Build history of the part. All positions in model axes, mm. A direction names the side the tool comes from. Round coordinates to 2 decimals unless told otherwise and drop trailing zeros. Write each loop counter-clockwise with the first axis right and the second up, starting at its lowest first coordinate (ties: lowest second). Pieces come first, ordered by that corner, then holes. Notation, with made-up numbers: (38.25, 2.25) -> (97.25, 2.25) arc R11 ccw to (97.25, 12.25) -> close; hole circle Ø11 at (20, 66). An arc over 180 degrees is marked (long way). One line per question, with ' | ' between items.
from build123d import *

# Parameters (mm, degrees)
F_3_6_3_6_DIAMETER_HOLE1_D     = 3.6
F_3_6_3_6_DIAMETER_HOLE1_DEPTH = 12
F_3_6_3_6_DIAMETER_HOLE1_TIP   = 1.081549114


with BuildPart() as part:
    # Sketch1 → Revolve1 (revolve)
    with BuildSketch(Plane.XY, mode=Mode.PRIVATE) as revolve1_sk:
        with BuildLine():
            Line((0, 14.67), (0, 5.5))
            Line((0, 5.5), (27, 5.5))
            Line((27, 5.5), (27, 11))
            ThreePointArc((27, 11), (22.050252532, 13.050252532), (20, 18))
            Line((20, 18), (20, 20))
            ThreePointArc((20, 20), (16, 24), (12, 20))
            Line((12, 20), (11, 20))
            Line((11, 20), (11, 13.17))
            Line((11, 13.17), (8, 13.17))
            Line((8, 13.17), (8, 14.67))
            Line((8, 14.67), (0, 14.67))
        make_face()
    revolve(revolve1_sk.sketch.rotate(Axis((0, 0, 0), (1, 0, 0)), 90), axis=Axis((0, 0, 0), (1, 0, 0)))

    # Ø3.6 (3.6) Diameter Hole1
    with Locations(Plane(origin=(21.47261693, 9.449479998, -9.92628458), x_dir=(0.49047083458, 0, 0.871457606787), z_dir=(0.789626152924, 0.423067471154, -0.444414731382))):
        with Locations((0, 0)):
            Hole(F_3_6_3_6_DIAMETER_HOLE1_D / 2, depth=F_3_6_3_6_DIAMETER_HOLE1_DEPTH)
            with Locations((0, 0, -(F_3_6_3_6_DIAMETER_HOLE1_DEPTH + F_3_6_3_6_DIAMETER_HOLE1_TIP / 2))):  # 118° drill point
                Cone(0, F_3_6_3_6_DIAMETER_HOLE1_D / 2, F_3_6_3_6_DIAMETER_HOLE1_TIP, mode=Mode.SUBTRACT)


solid = part.part
(1) Wall check: line 1 (Y direction, x = 16, z = 0); line 2 (Y direction, x = 7, z = 0); line 3 (X direction, y = 13.5, z = -5). Give the ranges that are in metal, low to high. Write a range as from..to.
Calculated:
line 1: -24..-5.5, 5.5..24 | line 2: -14.67..-5.5, 5.5..14.67 | line 3: 0..8, 11..21
(2) Slice it at A-A (z = 0). Write the cut outline in (x, y), then the cut area to 3 significant figures.
Calculated:
outline: (0, -14.67) -> (8, -14.67) -> (8, -13.17) -> (11, -13.17) -> (11, -20) -> (12, -20) arc R4 ccw to (20, -20) -> (20, -18) arc R7 cw to (27, -11) -> (27, -5.5) -> (0, -5.5) -> close; (0, 5.5) -> (27, 5.5) -> (27, 11) arc R7 cw to (20, 18) -> (20, 20) arc R4 ccw to (12, 20) -> (11, 20) -> (11, 13.17) -> (8, 13.17) -> (8, 14.67) -> (0, 14.67) -> close | area: 602 mm2
(3) Slice it at C-C (x = 2.5). Write the cut outline in (y, z).
Calculated:
outline: circle Ø29.34 at (0, 0); hole circle Ø11 at (0, 0)
(4) Slice it at D-D (x = 19). State how many separate pieces and enclosed holes the cut face has, then the cut area to 3 significant figures.
Calculated:
separate pieces: 1 | enclosed holes: 2 | area: 1,500 mm2
(5) Mould opens along Z. For faces 4 (the cylindrical face through (3.94, 8.93, -11.64)), 5 (the flat face through (11, 4, 13)), 6 (the conical face through (11.1, 4.17, -4.37)) say: pulls with the +Z half, pulls with the -Z half, needs draft (parallel to the pull), parting line crosses it, or undercut.
Calculated:
face 4: parting line crosses it | face 5: needs draft | face 6: undercut
(6) Drop flat-ended pins along their axis: pin 1 (6 mm diameter, centred on y = -9.5, z = -16, fed in from +X); pin 2 (1 mm diameter, centred on y = -11.5, z = 6, fed in from +X); pin 3 (1.5 mm diameter, centred on x = 23, z = -3.5, fed in from +Y); pin 4 (2 mm diameter, centred on y = 7, z = 4.5, fed in from -X). Give the stop position or say it passes through.
Calculated:
pin 1: x = 20.42 | pin 2: x = 22.71 | pin 3: y = 12.4 | pin 4: x = 0
(7) 3-axis set-ups, long thin cutter, end or side, ignore diameter. For faces 1 (the cylindrical face through (9.48, -3.96, 12.56)), 2 (the cylindrical face through (11.49, -0.88, -19.98)), 3 (the flat face through (20, -3, 18)): which of +Z, -Z, +X, -X, +Y, -Y reach the whole face in a straight line?
Calculated:
face 1: none | face 2: -X | face 3: +X
